```python
from build123d import *

# Parameters (mm, degrees)
BODY_MOVE_COPY1_ANGLE = 90


with BuildPart() as part:
    # Sketch1 → Revolve1 (revolve)
    with BuildSketch(Plane.XY, mode=Mode.PRIVATE) as revolve1_sk:
        Polygon((0, 4), (5.89, 4), (5.89, 9), (4.730911447, 9), (4.730911447, 23), (5.89, 23), (5.89, 26), (0, 26), align=None)
    revolve1 = revolve(revolve1_sk.sketch.rotate(Axis((0, 0, 0), (1, 0, 0)), 90), axis=Axis((0, 0, 0), (1, 0, 0)))

    # Sketch2 → Cut-Revolve1 (revolve, cut)
    with BuildSketch(Plane.XY, mode=Mode.PRIVATE) as cut_revolve1_sk:
        Polygon((0, 18), (1.977829822, 18), (4.889591697, 26), (0, 26), align=None)
    cut_revolve1 = revolve(cut_revolve1_sk.sketch.rotate(Axis((0, 0, 0), (1, 0, 0)), 90), axis=Axis((0, 0, 0), (1, 0, 0)), mode=Mode.SUBTRACT)

    # Mirror1: Revolve1, Cut-Revolve1 across Right Plane
    add(revolve1.mirror(Plane(origin=(0, 0, 0), x_dir=(0, 0, -1), z_dir=(1, 0, 0))))
    add(cut_revolve1.mirror(Plane(origin=(0, 0, 0), x_dir=(0, 0, -1), z_dir=(1, 0, 0))), mode=Mode.SUBTRACT)


with BuildPart() as part_1:
    # Body-Move/Copy1: moved
    add(part.part.rotate(Axis((0, 0, 0), (0, 1, 0)), BODY_MOVE_COPY1_ANGLE))


solid = part_1.part
```
Model file for the job. Use its own axes, mm. A direction names the side the tool comes from. Give positions to 0.01 mm unless a question says otherwise; leave off trailing zeros. Write each loop counter-clockwise with the first axis right and the second up, starting at its lowest first coordinate (ties: lowest second). Pieces come first, ordered by that corner, then holes. Notation, with made-up numbers: (38.5, 42.5) -> (44.5, 42.5) arc R22 ccw to (44.5, 77.5) -> close; hole circle Ø7 at (-38, 7.5). An arc over 180 degrees is marked (long way). Use CSV: the item, a comma, the result in double quotes. Start each with the question number.
1) Tool access for faces 1 (the conical face through (17.65, -5.56, -2.16)), 2 (the cylindrical face through (-2.994, -22.804, -5.319)), 3 (the flat face through (-10, 21, -5.89)), 4 (the flat face through (-10, 21, 5.89)), 5 (the flat face through (-10, 0, 4.731)): list every direction of +Z, -Z, +X, -X, +Y, -Y with a clear straight run to the whole face (end or side of a thin tool).
2) Two-plate mould, pull along X, no slides. Class faces 6 (the cylindrical face through (8.584, -2.703, -5.302)), 7 (the cylindrical face through (-20.633, 15.821, -5.383)), 8 (the flat face through (-2, 4, 5.89)): released by +X, released by -X, zero draft, split by the parting line, or undercut.
3) Cut at C-C on z = -2.75. List the corners of the cut face in (x, y).
4) Pin check, flat tips, straight feed: P1, Ø5, axis at x = 0, y = 0, coming from the -Z side; P2, Ø4, axis at x = -19.5, y = -8, coming from the +Z side; P3, Ø6, axis at x = 9.5, z = 2.5, coming from the -Y side; P4, Ø4, axis at x = 3, y = -15.5, coming from the +Z side. Stop position of each tip, or through.
5) Drill centre lines: L1, parallel to Y at x = 0, z = 5.3; L2, parallel to Y at x = -8, z = -5; L3, parallel to Z at x = 0.5, y = 12.5. Where is each one in solid material? Low to high.
Final values:
1,face 1,"none"
1,face 2,"-Z"
1,face 3,"-Z, +X, -X, +Y, -Y"
1,face 4,"+Z, +X, -X, +Y, -Y"
1,face 5,"+Z"
2,face 6,"undercut"
2,face 7,"split by the parting line"
2,face 8,"zero draft"
3,outline,"circle Ø40.24 at (0, 0); hole circle Ø8 at (0, 0)"
4,P1,"passes through"
4,P2,"stops at z = 5.89"
4,P3,"stops at y = -24.84"
4,P4,"stops at z = 4.73"
5,L1,"y = -26 to -23, -9 to -4, 4 to 9, 23 to 26"
5,L2,"y = -24.74 to -21.56, -4.12 to 4.12, 21.56 to 24.74"
5,L3,"z = -4.73 to 4.73"
